```python
from build123d import *

# Parameters (mm, degrees)
SKETCH1_W           = 90
SKETCH1_H           = 20
SKETCH1_R           = 2.65
SKETCH1_R_2         = 2.75
BOSS_EXTRUDE1_DEPTH = 20
CUT_EXTRUDE1_DEPTH  = 12
SKETCH3_R           = 5.5
CUT_EXTRUDE2_DEPTH  = 14
CHAMFER1_SIZE       = 3


with BuildPart() as part:
    # Sketch1 → Boss-Extrude1 (new body)
    with BuildSketch(Plane(origin=(0, 0, 0), x_dir=(1, 0, 0), z_dir=(0, 1, 0))):
        Rectangle(SKETCH1_W, SKETCH1_H)
        with Locations(Location((-21, 0, 0), (0, 0, 270))):
            Circle(SKETCH1_R, mode=Mode.SUBTRACT)
        with Locations(Location((21, 0, 0), (0, 0, 270))):
            Circle(SKETCH1_R, mode=Mode.SUBTRACT)
        with Locations(Location((-37, 0, 0), (0, 0, 270))):
            Circle(SKETCH1_R_2, mode=Mode.SUBTRACT)
        with Locations(Location((37, 0, 0), (0, 0, 270))):
            Circle(SKETCH1_R_2, mode=Mode.SUBTRACT)
    extrude(amount=BOSS_EXTRUDE1_DEPTH)

    # Sketch2 → Cut-Extrude1 (cut)
    with BuildSketch(Plane.XZ):
        Polygon((-16.265727793, 0), (-18.632863896, 4.1), (-23.367136104, 4.1), (-25.734272207, 0), (-23.367136104, -4.1), (-18.632863896, -4.1), align=None)
        Polygon((25.734272207, 0), (23.367136104, 4.1), (18.632863896, 4.1), (16.265727793, 0), (18.632863896, -4.1), (23.367136104, -4.1), align=None)
    extrude(amount=-CUT_EXTRUDE1_DEPTH, mode=Mode.SUBTRACT)

    # Sketch3 → Cut-Extrude2 (cut)
    with BuildSketch(Plane(origin=(0, 20, 0), x_dir=(1, 0, 0), z_dir=(0, 1, 0))):
        with Locations(Location((-37, 0, 0), (0, 0, 270))):
            Circle(SKETCH3_R)
        with Locations(Location((37, 0, 0), (0, 0, 270))):
            Circle(SKETCH3_R)
    extrude(amount=-CUT_EXTRUDE2_DEPTH, mode=Mode.SUBTRACT)

    # Chamfer1
    chamfer1_edges = [part.edges().sort_by_distance(p)[0] for p in [
        (45, 10, 10),
        (-45, 10, 10),
        (-45, 10, -10),
        (45, 10, -10),
    ]]
    chamfer(chamfer1_edges, length=CHAMFER1_SIZE)


solid = part.part
```
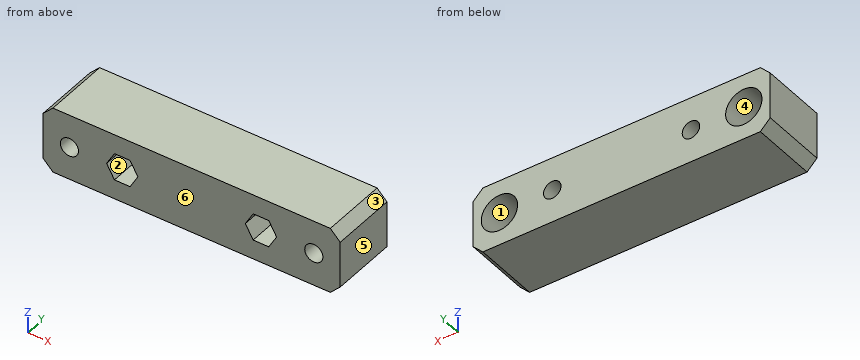
For this review, take the finished solid that the model builds, in its own axes (mm). Face numbers are marked on the shaded views. A direction names the side the tool comes from. Coordinates: 2 decimals unless noted, no trailing zeros. Order: outer loops, then holes, each group sorted by start corner. A loop starts at its lowest first (then second) coordinate and runs counter-clockwise, first axis right, second up. Notation, with made-up numbers: (-16, -32.5) - (33, -32.5) arc R23 cw to (33, 1.5) - close; hole circle Ø7 at (88.5, 9). An arc over 180 degrees is marked (long way). Answer as a JSON object with one key per item and string values. Group by question number.
1. We need section D-D on y = 16. State the section outline as (x, z) points, then the cut area to 3 significant figures.
2. We need section B-B on x = -37. State the section outline as (y, z) points.
3. We need section A-A on y = 2. State the section outline as (x, z) points.
4. The part is to be moulded in two halves that separate along X. For the marked faces 4, 5 and 6, say which applies: pulls with the +X half, pulls with the -X half, needs draft (parallel to the pull), parting line crosses it, or undercut.
5. Clearance check with flat-ended pins moving along their axes: P1, Ø6.5, axis at x = -37, z = 0, coming from the +Y side; P2, Ø4.5, axis at x = 37, z = 0, coming from the -Y side. State where each tip first meets the part, or that it passes through.
6. For probe 1 along X at (y, z) = (11.5, 0); probe 2 along X at (y, z) = (13.5, 0); probe 3 along Z at (x, y) = (21, 17), list the stretches that pass through material, from the lowest coordinate up.
7. We need section C-C on x = 21. State the section outline as (y, z) points.
8. For the marked faces 1, 2 and 3, list the 3-axis set-ups (+Z, -Z, +X, -X, +Y, -Y) from which the entire face can be reached by the end or side of a thin tool; tool diameter is ignored.
Final values:
{
 "1": {"outline": "(-45, -7) - (-42, -10) - (42, -10) - (45, -7) - (45, 7) - (42, 10) - (-42, 10) - (-45, 7) - close; hole circle Ø11 at (-37, 0); hole circle Ø5.3 at (-21, 0); hole circle Ø5.3 at (21, 0); hole circle Ø11 at (37, 0)", "area": "1,550 mm²"},
 "2": {"outline": "(0, -10) - (20, -10) - (20, -5.5) - (6, -5.5) - (6, -2.75) - (0, -2.75) - close; (0, 2.75) - (6, 2.75) - (6, 5.5) - (20, 5.5) - (20, 10) - (0, 10) - close"},
 "3": {"outline": "(-45, -7) - (-42, -10) - (42, -10) - (45, -7) - (45, 7) - (42, 10) - (-42, 10) - (-45, 7) - close; hole circle Ø5.5 at (-37, 0); hole (-25.73, 0) - (-23.37, -4.1) - (-18.63, -4.1) - (-16.27, 0) - (-18.63, 4.1) - (-23.37, 4.1) - close; hole (16.27, 0) - (18.63, -4.1) - (23.37, -4.1) - (25.73, 0) - (23.37, 4.1) - (18.63, 4.1) - close; hole circle Ø5.5 at (37, 0)"},
 "4": {"face 4": "undercut", "face 5": "pulls with the +X half", "face 6": "needs draft"},
 "5": {"P1": "y = 6", "P2": "through"},
 "6": {"probe 1": "-45 to -42.5, -31.5 to -25.73, -16.27 to 16.27, 25.73 to 31.5, 42.5 to 45", "probe 2": "-45 to -42.5, -31.5 to -23.65, -18.35 to 18.35, 23.65 to 31.5, 42.5 to 45", "probe 3": "-10 to -2.65, 2.65 to 10"},
 "7": {"outline": "(0, -10) - (20, -10) - (20, -2.65) - (12, -2.65) - (12, -4.1) - (0, -4.1) - close; (0, 4.1) - (12, 4.1) - (12, 2.65) - (20, 2.65) - (20, 10) - (0, 10) - close"},
 "8": {"face 1": "+Y", "face 2": "-Y", "face 3": "+Z, +X, +Y, -Y"}
}
